```python
from build123d import *

# Parameters (mm, degrees)
F1_DEPTH = 20


with BuildPart() as f1:
    # F0 (on Top) → F1 (new body)
    with BuildSketch(Plane.XY):
        with BuildLine():
            ThreePointArc((0, 6), (4.242641, 4.242641), (6, 0))
            Line((6, 0), (6, -19.25))
            ThreePointArc((6, -19.25), (6.21967, -19.78033), (6.75, -20))
            Line((6.75, -20), (8.6, -20))
            Line((8.6, -20), (8.6, 0))
            ThreePointArc((8.6, 0), (8.418451, 1.75775), (7.881468, 3.441287))
            ThreePointArc((7.881468, 3.441287), (7.616897, 5.784979), (8.718841, 7.870312))
            Line((8.718841, 7.870312), (24.060858, 23.21233))
            ThreePointArc((24.060858, 23.21233), (24.111472, 23.334524), (24.060858, 23.456718))
            Line((24.060858, 23.456718), (23.758788, 23.758788))
            Line((23.758788, 23.758788), (23.456718, 24.060858))
            ThreePointArc((23.456718, 24.060858), (23.334524, 24.111472), (23.21233, 24.060858))
            Line((23.21233, 24.060858), (7.870312, 8.718841))
            ThreePointArc((7.870312, 8.718841), (5.784979, 7.616897), (3.441287, 7.881468))
            ThreePointArc((3.441287, 7.881468), (1.75775, 8.418451), (0, 8.6))
            Line((0, 8.6), (-20, 8.6))
            Line((-20, 8.6), (-20, 6.75))
            ThreePointArc((-20, 6.75), (-19.78033, 6.21967), (-19.25, 6))
            Line((-19.25, 6), (0, 6))
        make_face()
    extrude(amount=F1_DEPTH)


solid = f1.part
```
Input: part model. Units: mm. Frame: model coordinates. A direction names the side the tool comes from. Give positions to 0.01 mm unless a question says otherwise; leave off trailing zeros. Loops run counter-clockwise (first coordinate to the right, second up) from the corner with the lowest first, then second, coordinate; pieces in that order, holes last.
1) Section query B-B on y = -8. Return the cut outline in (x, z), and give its area (3 significant figures).
A:
outline: (6, 0) - (8.6, 0) - (8.6, 20) - (6, 20) - close
area: 52.0 mm2
2) Line query: L1, parallel to X at y = -14.5, z = 5.25; L2, parallel to X at y = 1.5, z = 1.75. Output: solid intervals per line, ascending.
A:
L1: x = 6 to 8.6
L2: x = 5.81 to 8.47
3) Contact query for flat-ended pins moving along their axis: pin 1 (6 mm diameter, centred on y = 11, z = 6, fed in from -X); pin 2 (2 mm diameter, centred on y = -15, z = 13, fed in from +X); pin 3 (6 mm diameter, centred on x = -12, z = 10.5, fed in from +Y); pin 4 (6 mm diameter, centred on y = -9.5, z = 9, fed in from -X). Output: stop coordinate, or through.
A:
pin 1: stops at x = -20
pin 2: stops at x = 8.6
pin 3: stops at y = 8.6
pin 4: stops at x = 6
4) Section query A-A on z = 1.5. Return the cut outline in (x, y), and give its area (3 significant figures).
A:
outline: (-20, 6.75) arc R0.75 ccw to (-19.25, 6) - (0, 6) arc R6 cw to (6, 0) - (6, -19.25) arc R0.75 ccw to (6.75, -20) - (8.6, -20) - (8.6, 0) arc R8.6 ccw to (7.88, 3.44) arc R4 cw to (8.72, 7.87) - (24.06, 23.21) arc R0.17 ccw to (24.06, 23.46) - (23.46, 24.06) arc R0.17 ccw to (23.21, 24.06) - (7.87, 8.72) arc R4 cw to (3.44, 7.88) arc R8.6 ccw to (0, 8.6) - (-20, 8.6) - close
area: 167 mm2
5) Reachability of faces 1 (the flat face through (8.6, -10, 10)), 2 (the cylindrical face through (1.782, 8.413, 9.86)), 3 (the cylindrical face through (8.423, 1.733, 9.86)), 4 (the flat face through (-10, 8.6, 10)), 5 (the flat face through (-10, 6, 10)) from +Z, -Z, +X, -X, +Y, -Y: full face, straight path, thin tool, end or side. Return the list, or none.
A:
face 1: +Z, -Z, +X, -Y
face 2: +Z, -Z, +Y
face 3: +Z, -Z, +X
face 4: +Z, -Z, -X, +Y
face 5: +Z, -Z, -X, -Y
